```python
from build123d import *

# Parameters (mm, degrees)
ESQUISSE2_R             = 3
ENL_V_MAT_EXTRU_1_DEPTH = 164


with BuildPart() as part:
    # Esquisse1 → Révolution2 (revolve)
    with BuildSketch(Plane.XY, mode=Mode.PRIVATE) as r_volution2_sk:
        Polygon((0, 93.9493256), (77.14, 93.9493256), (77.14, 83.9493256), (59.3, 83.9493256), (59.3, 73.9493256), (59.3, 68.9493256), (55, 68.9493256), (55, 61.7493256), (59.3, 61.7493256), (59.3, 56.7493256), (55, 56.7493256), (55, 49.5493256), (59.3, 49.5493256), (59.3, 44.5493256), (55, 44.5493256), (55, 37.3493256), (59.3, 37.3493256), (59.3, 13.9493256), (55, 13.9493256), (0, 13.9493256), align=None)
    revolve(r_volution2_sk.sketch.rotate(Axis((0, 93.9493256, 0), (0, -1, 0)), 90), axis=Axis((0, 93.9493256, 0), (0, -1, 0)))  # turned: the seam where the file's is

    # Esquisse2 → Enlèv. mat.-Extru.1 (cut)
    with BuildSketch(Plane(origin=(0, 0, 0), x_dir=(1, 0, 0), z_dir=(0, 1, 0))):
        with Locations(Location((14.585474317, -69.42440161, 0), (0, 0, 90))):  # turned: the seam where the file's is
            Circle(ESQUISSE2_R)
        with Locations(Location((67.416032595, -22.080809521, 0), (0, 0, 90))):  # turned: the seam where the file's is
            Circle(ESQUISSE2_R)
        with Locations(Location((52.830558279, 47.34359209, 0), (0, 0, 90))):  # turned: the seam where the file's is
            Circle(ESQUISSE2_R)
        with Locations(Location((-14.585474317, 69.42440161, 0), (0, 0, 90))):  # turned: the seam where the file's is
            Circle(ESQUISSE2_R)
        with Locations(Location((-67.416032595, 22.080809521, 0), (0, 0, 90))):  # turned: the seam where the file's is
            Circle(ESQUISSE2_R)
        with Locations(Location((-52.830558279, -47.34359209, 0), (0, 0, 90))):  # turned: the seam where the file's is
            Circle(ESQUISSE2_R)
    extrude(amount=ENL_V_MAT_EXTRU_1_DEPTH, mode=Mode.SUBTRACT)


solid = part.part
```
CAD build for the part. Positions are in the model's coordinates, mm. A direction names the side the tool comes from. Round coordinates to 2 decimals unless told otherwise and drop trailing zeros. Write each loop counter-clockwise with the first axis right and the second up, starting at its lowest first coordinate (ties: lowest second). Pieces come first, ordered by that corner, then holes. Notation, with made-up numbers: (-30, 20) -> (13, 20) arc R13 cw to (13, 30) -> close; hole circle Ø7 at (25, 37). An arc over 180 degrees is marked (long way). Answer in a Markdown table with one row per item. Add a question column.
Item 1: Which spindle directions (+Z, -Z, +X, -X, +Y, -Y) get a long thin tool onto all of the face, cutting with end or side? Do faces 4 (the face through (45, 83.949, 40)), 5 (the face through (52.4, 68.949, 17.3)), 6 (the face through (-1, 13.949, 1)). Say none if no direction does.
Item 2: Drill centre lines: line 1 (Y direction, x = -46.5, z = -36.5); line 2 (Y direction, x = 56, z = 38.5); line 3 (X direction, y = 88, z = 70). Where is each one in solid material? Low to high. Write a range as from..to.
Item 3: Saw through at D-D, the plane y = 40. Write the cut outline in (x, z), then the cut area to 3 significant figures.
Item 4: Mould opens along Y. For faces 1 (the face through (-1, 93.949, 1)), 2 (the face through (-64.487, 88.879, -21.43)), 3 (the face through (48.794, 53.099, 25.379)) say: pulls with the +Y half, pulls with the -Y half, needs draft (parallel to the pull), parting line crosses it, or undercut.
Item 5: Drop flat-ended pins along their axis: pin 1 Ø5 at (x, z) = (14.59, 69.42) entering from +Y; pin 2 Ø10 at (x, y) = (-17, 53) entering from -Z; pin 3 Ø3 at (y, z) = (26.5, 24) entering from +X; pin 4 Ø4 at (y, z) = (23, -6.5) entering from -X. Give the stop position or say it passes through.
Item 6: Saw through at C-C, the plane y = 24.5. Write the cut outline in (x, z), then the cut area to 3 significant figures.
Findings below:
| question | item | result |
|---|---|---|
| 1 | face 4 | -Y |
| 1 | face 5 | none |
| 1 | face 6 | +Z, -Z, +X, -X, -Y |
| 2 | line 1 | y = 13.95..37.35, 44.55..49.55, 56.75..61.75, 68.95..93.95 |
| 2 | line 2 | y = 83.95..93.95 |
| 2 | line 3 | x = -32.41..11.64, 17.53..32.41 |
| 3 | outline | circle Ø110 at (0, 0) |
| 3 | area | 9,500 mm^2 |
| 4 | face 1 | pulls with the +Y half |
| 4 | face 2 | needs draft |
| 4 | face 3 | undercut |
| 5 | pin 1 | passes through |
| 5 | pin 2 | stops at z = -57.77 |
| 5 | pin 3 | stops at x = 54.87 |
| 5 | pin 4 | stops at x = -59.13 |
| 6 | outline | circle Ø118.6 at (0, 0) |
| 6 | area | 11,000 mm^2 |
